Geometry check sheet. Reference: the model listing, model coordinates, mm. A direction names the side the tool comes from. Give positions to 0.01 mm unless a question says otherwise; leave off trailing zeros. Write each loop counter-clockwise with the first axis right and the second up, starting at its lowest first coordinate (ties: lowest second). Pieces come first, ordered by that corner, then holes. Notation, with made-up numbers: M 58.25,30.25 L 116.25,30.25 A21 ccw 116.25,41.25 Z; hole C 81,1 d11. An arc over 180 degrees is marked long. One line per item, written item: value. Start each with the question number.
1. Scan lines: line 1 (Z direction, x = 15, y = -6); line 2 (Y direction, x = 32, z = 4); line 3 (Z direction, x = 20.5, y = -63.5) (3 decimals). Record each from-to range of solid material in increasing order.
2. Release check for a two-part mould opening along X. For faces 1 (the face through (37.15, -75.29, 8.49)), 2 (the face through (19.317, -38.91, -0.873)), 3 (the face through (0, -38, 1)), 4 (the face through (11.08, -69.66, 8.52)) record: pulls with the +X half, pulls with the -X half, needs draft (parallel to the pull), parting line crosses it, or undercut.
3. Cross-section at D-D on z = 8.25. Count the separate pieces of the cut face and the enclosed holes in it, then the cut area to 3 significant figures.
4. Gauge pin test, flat ends, axial feed: pin 1 (3 mm diameter, centred on x = 7, y = -55, fed in from -Z); pin 2 (4 mm diameter, centred on x = 17.5, z = 3.5, fed in from +Y); pin 3 (6 mm diameter, centred on x = 20.5, z = 0.5, fed in from +Y); pin 4 (2 mm diameter, centred on x = 8.5, z = 4.5, fed in from -Y). Record the tip position at first contact, or that the pin passes through.
5. Cross-section at B-B on y = -46. Record the cut outline in (x, z) (3 decimals), then the cut area to 3 significant figures.
6. Cross-section at A-A on x = 27.5. Record the cut outline in (y, z) (3 decimals).
7. Cross-section at C-C on x = 5. Record the cut outline in (y, z) (3 decimals).
8. Tool access check on faces 5 (the face through (38.1, -38, 1)), 6 (the face through (19, -38.1, 4)), 7 (the face through (19, -59, 7.493)). Record the directions out of +Z, -Z, +X, -X, +Y, -Y that give a thin tool (end or side, any length) a straight path to the whole face; none if there is none.
from build123d import *

# Parameters (mm, degrees)
BOSS_EXTRUDE1_DEPTH = 38.1
FILLET1_R           = 2.032
FILLET2_R           = 4.064
FILLET3_R           = 3.175
SKETCH2_R           = 3.3655
CUT_EXTRUDE1_DEPTH  = 12.557


with BuildPart() as part:
    # Sketch1 → Boss-Extrude1 (new body)
    with BuildSketch(Plane(origin=(0, 0, 0), x_dir=(0, 0, -1), z_dir=(1, 0, 0))):
        Polygon((0, 0), (0, -38.1), (-9.525, -38.1), (-9.525, -76.2), (-7.493, -76.2), (-7.493, -40.132), (2.032, -40.132), (2.032, 0), align=None)
    extrude(amount=BOSS_EXTRUDE1_DEPTH)

    # Fillet1
    fillet1_edges = [part.edges().sort_by_distance(p)[0] for p in [
        (19.05, -40.132, 7.493),
        (19.05, -38.1, 0),
    ]]
    fillet(fillet1_edges, radius=FILLET1_R)

    # Fillet2
    fillet2_edges = [part.edges().sort_by_distance(p)[0] for p in [
        (19.05, -40.132, -2.032),
        (19.05, -38.1, 9.525),
    ]]
    fillet(fillet2_edges, radius=FILLET2_R)

    # Fillet3
    fillet3_edges = [part.edges().sort_by_distance(p)[0] for p in [
        (0, 0, -1.016),
        (38.1, -76.2, 8.509),
        (38.1, 0, -1.016),
        (0, -76.2, 8.509),
    ]]
    fillet(fillet3_edges, radius=FILLET3_R)

    # Sketch2 → Cut-Extrude1 (cut, through all)
    with BuildSketch(Plane.XY.offset(9.525)):
        with Locations((9.525, -66.675)):
            Circle(SKETCH2_R)
        with Locations((28.575, -47.625)):
            Circle(SKETCH2_R)
    extrude(amount=-CUT_EXTRUDE1_DEPTH, mode=Mode.SUBTRACT)


solid = part.part
Report:
1. line 1: z = -2.03 to 0
1. line 2: y = -40.13 to -38.1
1. line 3: z = 7.493 to 9.525
2. face 1: pulls with the +X half
2. face 2: needs draft
2. face 3: pulls with the -X half
2. face 4: undercut
3. separate pieces: 1
3. enclosed holes: 2
3. area: 1,330 mm^2
4. pin 1: stops at z = 7.49
4. pin 2: stops at y = -38.03
4. pin 3: stops at y = 0
4. pin 4: stops at y = -40.13
5. outline: M 0,7.493 L 25.628,7.493 L 25.628,9.525 L 0,9.525 Z; M 31.522,7.493 L 38.1,7.493 L 38.1,9.525 L 31.522,9.525 Z
5. area: 65.4 mm^2
6. outline: M -76.2,7.493 L -50.814,7.493 L -50.814,9.525 L -76.2,9.525 Z; M -44.436,7.493 L -42.164,7.493 A2.032 cw -40.132,5.461 L -40.132,2.032 A4.064 ccw -36.068,-2.032 L 0,-2.032 L 0,0 L -36.068,0 A2.032 cw -38.1,2.032 L -38.1,5.461 A4.064 ccw -42.164,9.525 L -44.436,9.525 Z
7. outline: M -76.2,7.493 L -42.164,7.493 A2.032 cw -40.132,5.461 L -40.132,2.032 A4.064 ccw -36.068,-2.032 L 0,-2.032 L 0,0 L -36.068,0 A2.032 cw -38.1,2.032 L -38.1,5.461 A4.064 ccw -42.164,9.525 L -76.2,9.525 Z
8. face 5: +Z, -Z, +X, +Y, -Y
8. face 6: +Z, +X, -X, +Y
8. face 7: -Z, +X, -X, -Y
